```python
from build123d import *

# Parameters (mm, degrees)
F0_R     = 6.5
F0_R_2   = 5
F0_R_3   = 1.5
F1_DEPTH = 3
F2_DEPTH = 3.55
F3_DEPTH = 3.45
F4_W     = 3
F4_H     = 0.75
F4_W_2   = 0.75
F4_H_2   = 3
F5_DEPTH = 0.45


with BuildPart() as f1:
    # F0 (on Right) → F1 (new body)
    with BuildSketch(Plane.YZ):
        Circle(F0_R)
        Circle(F0_R_2, mode=Mode.SUBTRACT)
        Circle(F0_R_2)
        Circle(F0_R_3, mode=Mode.SUBTRACT)
        Circle(F0_R_3)
    extrude(amount=F1_DEPTH)

    # F0 (on Right) → F2 (join)
    with BuildSketch(Plane.YZ):
        Circle(F0_R_2)
        Circle(F0_R_3, mode=Mode.SUBTRACT)
    extrude(amount=F2_DEPTH)

    # F0 (on Right) → F3 (join)
    with BuildSketch(Plane.YZ):
        Circle(F0_R_3)
    extrude(amount=F3_DEPTH)

    # F4 (on face) → F5 (join, through all)
    with BuildSketch(Plane.YZ.offset(3.45)):
        with Locations((0, 5.625)):
            Rectangle(F4_W, F4_H)
        Polygon((5.303301, 3.181981), (3.181981, 5.303301), (2.65165, 4.772971), (4.772971, 2.65165), align=None)
        with Locations((5.625, 0)):
            Rectangle(F4_W_2, F4_H_2)
        Polygon((3.181981, -5.303301), (5.303301, -3.181981), (4.772971, -2.65165), (2.65165, -4.772971), align=None)
        with Locations((0, -5.625)):
            Rectangle(F4_W, F4_H)
        Polygon((-5.303301, -3.181981), (-3.181981, -5.303301), (-2.65165, -4.772971), (-4.772971, -2.65165), align=None)
        with Locations((-5.625, 0)):
            Rectangle(F4_W_2, F4_H_2)
        Polygon((-3.181981, 5.303301), (-5.303301, 3.181981), (-4.772971, 2.65165), (-2.65165, 4.772971), align=None)
    extrude(amount=-F5_DEPTH)


solid = f1.part
```
Geometry check sheet. Reference: the model listing, model coordinates, mm. A direction names the side the tool comes from. Coordinates: 2 decimals unless noted, no trailing zeros. Order: outer loops, then holes, each group sorted by start corner. A loop starts at its lowest first (then second) coordinate and runs counter-clockwise, first axis right, second up. Notation, with made-up numbers: M 13.5,-20.75 L 43.5,-20.75 A27 cw 43.5,17.25 Z; hole C -4,46 d4. An arc over 180 degrees is marked long. One line per question, with ' | ' between items. Start each with the question number.
Item 1: Gauge pin test, flat ends, axial feed: pin 1 (0.5 mm diameter, centred on x = 3, y = -5.5, fed in from -Z); pin 2 (0.5 mm diameter, centred on x = 3, z = 0.5, fed in from -Y); pin 3 (0.5 mm diameter, centred on x = 3.5, z = 5.5, fed in from +Y); pin 4 (6 mm diameter, centred on y = 0.5, z = -0.5, fed in from +X). Record the tip position at first contact, or that the pin passes through.
Item 2: Cross-section at D-D on y = 1.75. Enter the section's corners in (x, z), then the cut area to 3 significant figures.
Item 3: Material ranges on L1, parallel to Z at x = 3.5, y = 0; L2, parallel to Y at x = 3.1, z = 0; L3, parallel to X at y = 3, z = -5.5, recorded low to high. Write a range as [from, to].
Item 4: Draft check along Y on faces 1 (the flat face through (3.228, 3.727, -3.697)), 2 (the flat face through (3.45, 4, 4)), 3 (the cylindrical face through (1.479, -5.158, -3.955)). Enter one of: pulls with the +Y half, pulls with the -Y half, needs draft (parallel to the pull), parting line crosses it, or undercut.
Item 5: Set-up check for faces 4 (the flat face through (3.45, -4, -4)), 5 (the flat face through (3.228, -3.697, -3.727)), 6 (the flat face through (3.228, -4.228, 4.257)), 7 (the flat face through (3.45, 4, -4)): record each of +Z, -Z, +X, -X, +Y, -Y from which the full face is reachable in a straight line by a thin tool's end or side.
Item 6: Cross-section at A-A on y = 0. Enter the section's corners in (x, z).
Item 7: Cross-section at C-C on x = 1.15. Enter the section's corners in (y, z).
Findings:
1) pin 1: stops at z = -3.83 | pin 2: stops at y = -6.5 | pin 3: stops at y = 3.23 | pin 4: stops at x = 3.55
2) outline: M 0,-6.26 L 3,-6.26 L 3,-4.68 L 3.55,-4.68 L 3.55,4.68 L 3,4.68 L 3,6.26 L 0,6.26 Z | area: 42.7 mm²
3) L1: z = [-5, -1.5], [1.5, 5] | L2: y = [-6, -5.25], [-5, 5], [5.25, 6] | L3: x = [0, 3]
4) face 1: undercut | face 2: needs draft | face 3: parting line crosses it
5) face 4: -Z, +X, -Y | face 5: +X | face 6: +Z, +X, -Y | face 7: -Z, +X, +Y
6) outline: M 0,-6.5 L 3,-6.5 L 3,-6 L 3.45,-6 L 3.45,-5.25 L 3,-5.25 L 3,-5 L 3.55,-5 L 3.55,-1.5 L 3.45,-1.5 L 3.45,1.5 L 3.55,1.5 L 3.55,5 L 3,5 L 3,5.25 L 3.45,5.25 L 3.45,6 L 3,6 L 3,6.5 L 0,6.5 Z
7) outline: C 0,0 d13
